Answer from the drawing. Dimensions are ordinates in mm from the lowest x, y and z of the part. Coordinates: 2 decimals unless noted, no trailing zeros. Order: outer loops, then holes, each group sorted by start corner. A loop starts at its lowest first (then second) coordinate and runs counter-clockwise, first axis right, second up. Notation, with made-up numbers: M -29.75,-32.5 L -2.75,-32.5 A24 ccw -2.75,3.5 Z; hole C 64,23.5 d6. An arc over 180 degrees is marked long. One line per question, with ' | ' between items. Start each with the question number.
1) Given P1, Ø1.5, axis at x = 2, y = 152.5, coming from the -Z side; P2, Ø1.5, axis at x = 2, z = 2, coming from the +Y side; P3, Ø0.9, axis at x = 2, z = 54, coming from the +Y side, each flat-ended and moving along its own axis, determine where each tip first touches the part or whether it passes through.
2) Find section C-C, the plane z = 67.5. Write down the section's boundary in (x, y), plus the area to 3 significant figures.
3) Consider probe 1 along Y at (x, z) = (2.7, 59); probe 2 along Z at (x, y) = (2.6, 43.5); probe 3 along Y at (x, z) = (1.45, 152.5). Determine where each line is inside the solid, lowest interval first.
4) Find section B-B, the plane y = 38. Write down the section's boundary in (x, z).
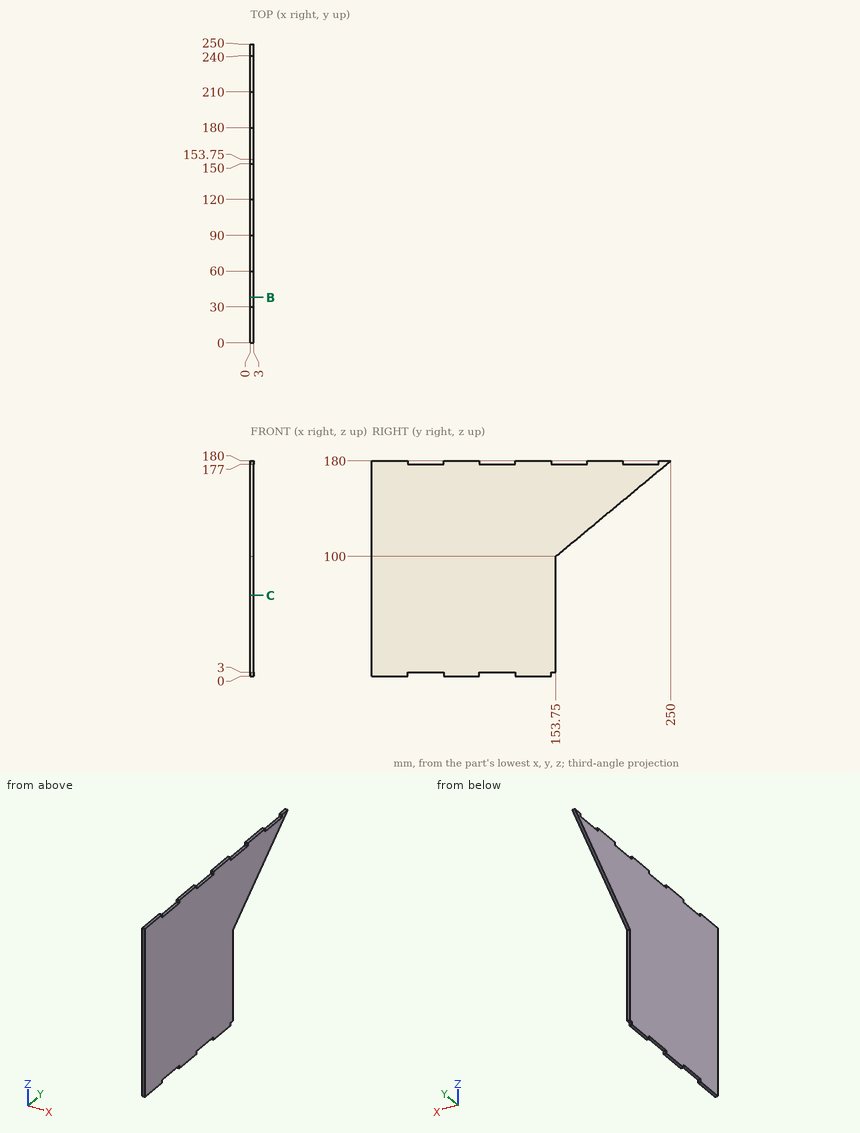
Report:
1) P1: stops at z = 3 | P2: stops at y = 150 | P3: stops at y = 153.75
2) outline: M 0,0 L 3,0 L 3,153.75 L 0,153.75 Z | area: 461 mm^2
3) probe 1: y = 0 to 153.75 | probe 2: z = 3 to 177 | probe 3: y = 0 to 216.91
4) outline: M 0,3 L 3,3 L 3,177 L 0,177 Z
